Source: CAD feature listing. Evaluate the final solid. Frame: model axes, mm. Face numbers are marked on the shaded views. A direction names the side the tool comes from. Give positions to 0.01 mm unless a question says otherwise; leave off trailing zeros. Order: outer loops, then holes, each group sorted by start corner. A loop starts at its lowest first (then second) coordinate and runs counter-clockwise, first axis right, second up.
1) Material intervals for line 1 (Y direction, x = 13.25, z = 0.4); line 2 (X direction, y = 31, z = 0.5) (3 decimals); line 3 (Y direction, x = 2.5, z = 1.55) (3 decimals), sorted ascending.
2) Section D-D, the plane y = 31. Return loops of the section in (x, z) (3 decimals), plus the area to 3 significant figures.
3) Access query for the marked faces 1 and 2. Directions: +Z, -Z, +X, -X, +Y, -Y. A direction counts if a zero-diameter tool reaches every point of the face in a straight line with its end or side. Return the directions, or none.
4) Section A-A, the plane x = 6. Return loops of the section in (y, z).
5) Section B-B, the plane y = 49. Return loops of the section in (x, z), plus the area to 3 significant figures.
6) Draft query along Y for the marked faces 3, 4 and 5. Return one class per face: released by +Y, released by -Y, zero draft, split by the parting line, or undercut.
7) Section C-C, the plane z = 2.15. Give the number of separate pieces and of enclosed holes in the cut face, plus the area to 3 significant figures.
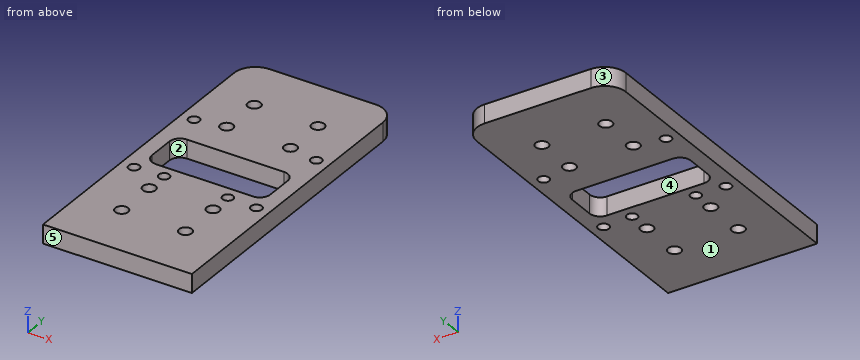
```python
from build123d import *

# Parameters (mm, degrees)
BOSS_EXTRU_1_DEPTH      = 3.5
ESQUISSE2_R             = 1.2
ESQUISSE2_R_2           = 1.025
ENL_V_MAT_EXTRU_1_DEPTH = 66.852107028
ENL_V_MAT_EXTRU_2_DEPTH = 66.852107028
ESQUISSE7_R             = 1
ENL_V_MAT_EXTRU_4_DEPTH = 66.852107028


with BuildPart() as part:
    # Esquisse1 → Boss.-Extru.1 (new body)
    with BuildSketch(Plane.XY):
        with BuildLine():
            Line((0, 0), (28, 0))
            Line((28, 0), (28, 55.5))
            ThreePointArc((28, 55.5), (26.828427125, 58.328427125), (24, 59.5))
            Line((24, 59.5), (4, 59.5))
            ThreePointArc((4, 59.5), (1.171572875, 58.328427125), (0, 55.5))
            Line((0, 55.5), (0, 0))
        make_face()
    extrude(amount=BOSS_EXTRU_1_DEPTH)

    # Esquisse2 → Enlèv. mat.-Extru.1 (cut, through all)
    with BuildSketch(Plane.XY.offset(3.5)):
        with Locations((8, 10.5)):
            Circle(ESQUISSE2_R)
        with Locations((20, 10.5)):
            Circle(ESQUISSE2_R)
        with Locations((8, 18.5)):
            Circle(ESQUISSE2_R)
        with Locations((20, 18.5)):
            Circle(ESQUISSE2_R)
        with Locations((8, 49)):
            Circle(ESQUISSE2_R)
        with Locations((8, 41)):
            Circle(ESQUISSE2_R)
        with Locations((20, 49)):
            Circle(ESQUISSE2_R)
        with Locations((20, 41)):
            Circle(ESQUISSE2_R)
        with Locations((2.5, 40)):
            Circle(ESQUISSE2_R_2)
        with Locations((2.5, 22.6)):
            Circle(ESQUISSE2_R_2)
        with Locations((25.5, 40)):
            Circle(ESQUISSE2_R_2)
        with Locations((25.5, 22.6)):
            Circle(ESQUISSE2_R_2)
    extrude(amount=-ENL_V_MAT_EXTRU_1_DEPTH, mode=Mode.SUBTRACT)

    # Esquisse3 → Enlèv. mat.-Extru.2 (cut, through all)
    with BuildSketch(Plane.XY.offset(3.5)):
        with BuildLine():
            Line((4.875, 34.25), (23.125, 34.25))
            ThreePointArc((23.125, 34.25), (24.539213562, 33.664213562), (25.125, 32.25))
            Line((25.125, 32.25), (25.125, 27.25))
            ThreePointArc((25.125, 27.25), (24.539213562, 25.835786438), (23.125, 25.25))
            Line((23.125, 25.25), (4.875, 25.25))
            ThreePointArc((4.875, 25.25), (3.460786438, 25.835786438), (2.875, 27.25))
            Line((2.875, 27.25), (2.875, 32.25))
            ThreePointArc((2.875, 32.25), (3.460786438, 33.664213562), (4.875, 34.25))
        make_face()
    extrude(amount=-ENL_V_MAT_EXTRU_2_DEPTH, mode=Mode.SUBTRACT)

    # Esquisse7 → Enlèv. mat.-Extru.4 (cut, through all)
    with BuildSketch(Plane.XY.offset(3.5)):
        with Locations((8, 22.82)):
            Circle(ESQUISSE7_R)
        with Locations((20, 22.82)):
            Circle(ESQUISSE7_R)
    extrude(amount=-ENL_V_MAT_EXTRU_4_DEPTH, mode=Mode.SUBTRACT)


solid = part.part
```
From the geometry:
1. line 1: y = 0 to 25.25, 34.25 to 59.5
1. line 2: x = 0 to 2.875, 25.125 to 28
1. line 3: y = 0 to 21.575, 23.625 to 38.975, 41.025 to 59.208
2. outline: (0, 0) - (2.875, 0) - (2.875, 3.5) - (0, 3.5) - close; (25.125, 0) - (28, 0) - (28, 3.5) - (25.125, 3.5) - close
2. area: 20.1 mm2
3. face 1: -Z, +X, -X, +Y, -Y
3. face 2: +Z, -Z
4. outline: (0, 0) - (25.25, 0) - (25.25, 3.5) - (0, 3.5) - close; (34.25, 0) - (59.5, 0) - (59.5, 3.5) - (34.25, 3.5) - close
5. outline: (0, 0) - (6.8, 0) - (6.8, 3.5) - (0, 3.5) - close; (9.2, 0) - (18.8, 0) - (18.8, 3.5) - (9.2, 3.5) - close; (21.2, 0) - (28, 0) - (28, 3.5) - (21.2, 3.5) - close
5. area: 81.2 mm2
6. face 3: released by +Y
6. face 4: undercut
6. face 5: released by -Y
7. separate pieces: 1
7. enclosed holes: 15
7. area: 1,410 mm2
